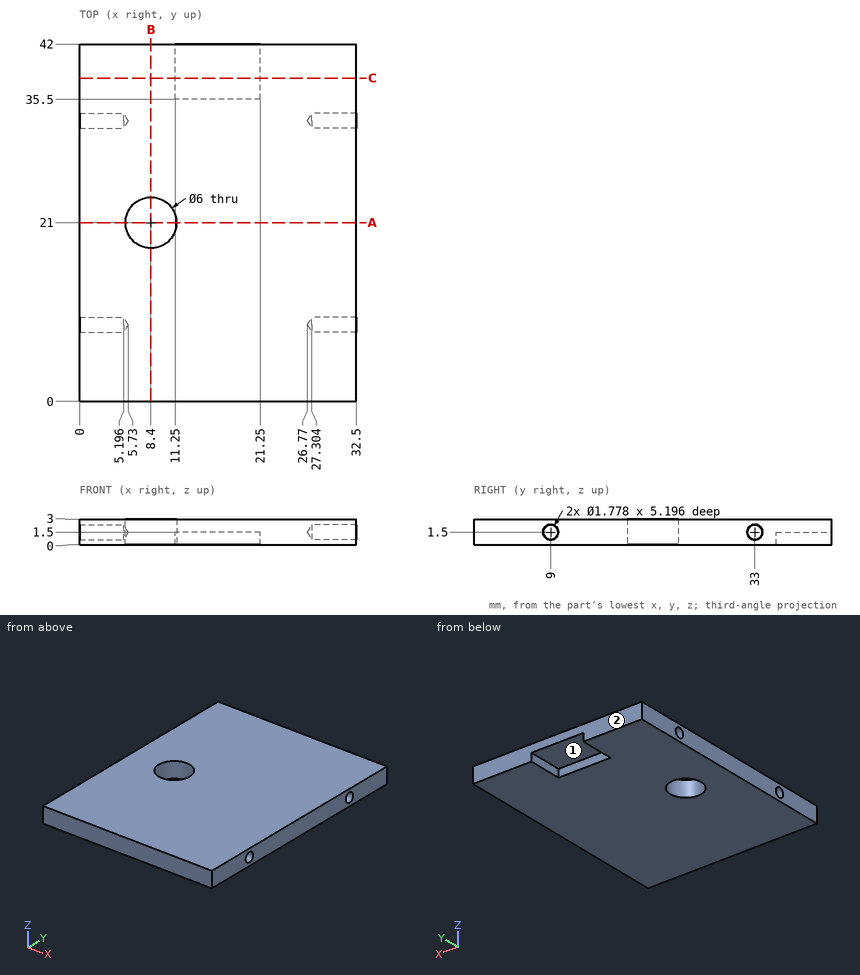
Source: three-view drawing plus pictorial views. Frame: mm from the lowest corner of the part. Round coordinates to 2 decimals unless told otherwise and drop trailing zeros. Write each loop counter-clockwise with the first axis right and the second up, starting at its lowest first coordinate (ties: lowest second). Pieces come first, ordered by that corner, then holes. Notation, with made-up numbers: M 67,13 L 79,13 A25 ccw 79,50 Z; hole C 41,24 d7. An arc over 180 degrees is marked long. Write item = value, one per line.
Item 1: Pin query (flat end, axial travel): P1, Ø0.8, axis at x = 15.5, z = 1, coming from the +Y side; P2, Ø1.1, axis at y = 9, z = 1.5, coming from the +X side; P3, Ø1.6, axis at y = 33, z = 1.5, coming from the -X side. Return the tip coordinate at first contact, or that it passes through.
Findings:
P1 = 35.5
P2 = 27.1
P3 = 5.25
Item 2: Section query C-C on y = 38. Return loops of the section in (x, z).
Findings:
outline = M 0,0 L 11.25,0 L 11.25,1.5 L 21.25,1.5 L 21.25,0 L 32.5,0 L 32.5,3 L 0,3 Z
Item 3: Section query A-A on y = 21. Return loops of the section in (x, z), then the cut area to 3 significant figures.
Findings:
outline = M 0,0 L 5.4,0 L 5.4,3 L 0,3 Z; M 11.4,0 L 32.5,0 L 32.5,3 L 11.4,3 Z
area = 79.5 mm^2
Item 4: Material intervals for line 1 along Y through (x, z) = (2.1, 1.5); line 2 along X through (y, z) = (39, 1.2); line 3 along Z through (x, y) = (28.55, 33), sorted ascending. Write a range as [from, to].
Findings:
line_1 = [0, 8.11], [9.89, 32.11], [33.89, 42]
line_2 = [0, 11.25], [21.25, 32.5]
line_3 = [0, 0.61], [2.39, 3]
Item 5: Pull-direction query (X, two-part tool) for the marked faces 1 and 2; classes: pulls with the +X half, pulls with the -X half, needs draft (parallel to the pull), parting line crosses it, or undercut.
Findings:
face_1 = undercut
face_2 = needs draft
Item 6: Section query B-B on x = 8.4. Return loops of the section in (y, z), then the cut area to 3 significant figures.
Findings:
outline = M 0,0 L 18,0 L 18,3 L 0,3 Z; M 24,0 L 42,0 L 42,3 L 24,3 Z
area = 108 mm^2
